Check sheet for the drawn part. Datum: minimum x, y, z corner. Units: mm. Give positions to 0.01 mm unless a question says otherwise; leave off trailing zeros. Order: outer loops, then holes, each group sorted by start corner. A loop starts at its lowest first (then second) coordinate and runs counter-clockwise, first axis right, second up. Notation, with made-up numbers: (67, 84.5) -> (76, 84.5) arc R22 ccw to (76, 115.5) -> close; hole circle Ø4 at (51.5, -4.75). An arc over 180 degrees is marked (long way). One line per question, with ' | ' between items. Start each with the question number.
Q1. Section check A-A on y = 0.9. Give the number of separate pieces and of enclosed holes in the cut face, plus the area to 3 significant figures.
Q2. Section check B-B on x = 10.5. Record the cut outline in (y, z).
Q3. Go/stop test with flat-tipped pins: pin 1 (5 mm diameter, centred on x = 4, z = 130.5, fed in from -Y); pin 2 (1 mm diameter, centred on y = 0.5, z = 78, fed in from -X). Record where each tip stops, or that it passes through.
Q4. Material ranges on probe 1 along Z at (x, y) = (7.75, 1.75); probe 2 along X at (y, z) = (0.55, 20); probe 3 along Z at (x, y) = (6.5, 1.2), recorded low to high. Write a range as [from, to].
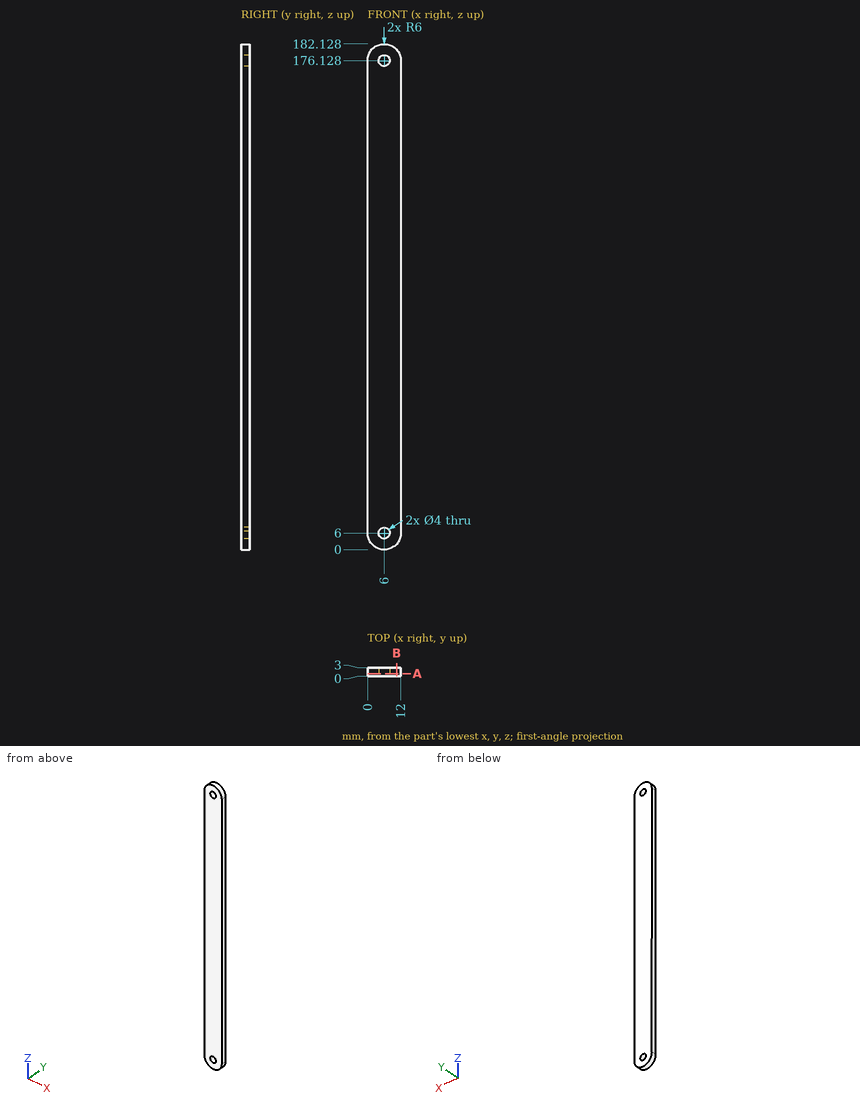
Filled in:
1) separate pieces: 1 | enclosed holes: 2 | area: 2,130 mm²
2) outline: (0, 2.03) -> (3, 2.03) -> (3, 180.1) -> (0, 180.1) -> close
3) pin 1: y = 0 | pin 2: x = 0.02
4) probe 1: [0.26, 5.03], [6.97, 175.16], [177.1, 181.87] | probe 2: [0.03, 12] | probe 3: [0.02, 4.06], [7.94, 174.19], [178.06, 182.11]
